Drawing for the job (mm, zero at the part's lowest x, y, z). Coordinates: 2 decimals unless noted, no trailing zeros. Loops run counter-clockwise (first coordinate to the right, second up) from the corner with the lowest first, then second, coordinate; pieces in that order, holes last. Notation, with made-up numbers: (87, 62) -> (137, 62) arc R17 cw to (137, 73) -> close; hole circle Ø10 at (78.25, -30.75). An arc over 180 degrees is marked (long way). Write item = value, one per line. Start each with the question number.
(1) Band-saw the part on B-B (y = 95). Write the cut outline in (x, z).
(2) Flat gauge pins, fed straight in: P1, Ø1.5, axis at x = 268, y = 104, coming from the -Z side; P2, Ø12, axis at x = 483.5, z = 634, coming from the -Y side. Where does each tip first touch, or does it go through?
(3) Band-saw the part on A-A (z = 111). Write the cut outline in (x, y).
(4) Pull direction X, two halves, no side cores. Call the marked faces 1 and 2: +X half, -X half, draft (parallel to the pull), parting line (faces both ways), or undercut.
(5) Drill centre line: line 1 (Z direction, x = 34.5, y = 277). Where is it in solid material? Low to high. Write a range as from..to.
(6) Band-saw the part on C-C (x = 339.5). Write the cut outline in (y, z), and give its area (3 significant figures).
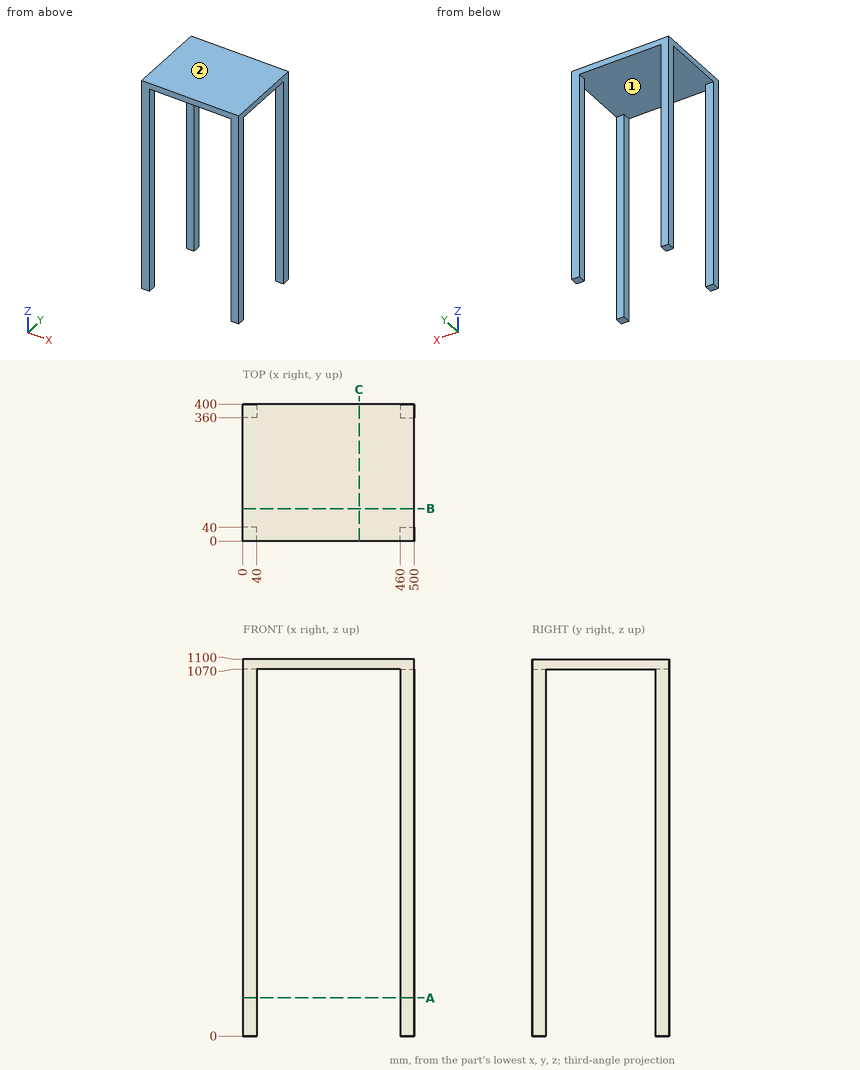
Findings below:
q1.outline = (0, 1070) -> (500, 1070) -> (500, 1100) -> (0, 1100) -> close
q2.P1 = 1070
q2.P2 = 0
q3.outline = (0, 0) -> (40, 0) -> (40, 40) -> (0, 40) -> close; (0, 360) -> (40, 360) -> (40, 400) -> (0, 400) -> close; (460, 0) -> (500, 0) -> (500, 40) -> (460, 40) -> close; (460, 360) -> (500, 360) -> (500, 400) -> (460, 400) -> close
q4.face_1 = undercut
q4.face_2 = draft
q5.line_1 = 1070..1100
q6.outline = (0, 1070) -> (400, 1070) -> (400, 1100) -> (0, 1100) -> close
q6.area = 12,000 mm²
